Can you work these out from the model? Positions are in its coordinate system, mm. A direction names the side the tool comes from. Coordinates: 2 decimals unless noted, no trailing zeros. Loops run counter-clockwise (first coordinate to the right, second up) from the corner with the lowest first, then second, coordinate; pieces in that order, holes last. Notation, with made-up numbers: (57.25, 1) -> (96.25, 1) arc R20 cw to (96.25, 18) -> close; hole circle Ø5 at (67.5, -1.5). An arc over 180 degrees is marked (long way). Put each result on its own line as item: value. Start each with the question number.
Item 1: We'd pull the mould along Z, two halves only. Please class faces 1 (the flat face through (0, 11, -20.5)), 2 (the cylindrical face through (-41, -73.95, 21.07)), 3 (the cylindrical face through (-41.07, -73.95, -21)): pulls with the +Z half, pulls with the -Z half, needs draft (parallel to the pull), parting line crosses it, or undercut.
Item 2: Will these pins go through, and if not, where does the flat tip stop? P1, Ø0.6, axis at x = 2.5, z = -21, coming from the +Y side; P2, Ø0.6, axis at y = -153.5, z = -21.5, coming from the +X side; P3, Ø22.5, axis at x = 12.5, z = 8, coming from the -Y side.
Item 3: If we section it at B-B on x = -33: Please give me the cut outline in (y, z), plus the area to 3 significant figures.
Item 4: If we section it at D-D on z = -15.5: Please give me the cut outline in (x, y).
Item 5: Please list where these lines run through material, in increasing order: L1, parallel to X at y = -157.5, z = -21.65; L2, parallel to Y at x = 0, z = -21.8; L3, parallel to Y at x = 4, z = 14.5. Write a range as from..to.
Item 6: If we section it at A-A on x = 0: Please give me the cut outline in (y, z), plus the area to 3 significant figures.
Item 7: If we section it at C-C on z = 4: Please give me the cut outline in (x, y).
Item 8: For faces 4 (the cylindrical face through (-5.46, 12.32, 7)), 5 (the flat face through (0, -161, -20.5)), 6 (the flat face through (-1, -76, -22.5)), which set-ups out of +Z, -Z, +X, -X, +Y, -Y let a thin tool reach every point of the face, with its end or its side?
```python
from build123d import *

# Parameters (mm, degrees)
F1_DEPTH = 150
F2_R     = 3
F3_DEPTH = 2
F4_R     = 10
F5_DEPTH = 25


with BuildPart() as f1:
    # F0 (on Front) → F1 (new body)
    with BuildSketch(Plane.XZ):
        with BuildLine():
            ThreePointArc((42.5, 17.5), (41.035534, 21.035534), (37.5, 22.5))
            Line((37.5, 22.5), (-37.5, 22.5))
            ThreePointArc((-37.5, 22.5), (-41.035534, 21.035534), (-42.5, 17.5))
            Line((-42.5, 17.5), (-42.5, -17.5))
            ThreePointArc((-42.5, -17.5), (-41.035534, -21.035534), (-37.5, -22.5))
            Line((-37.5, -22.5), (37.5, -22.5))
            ThreePointArc((37.5, -22.5), (41.035534, -21.035534), (42.5, -17.5))
            Line((42.5, -17.5), (42.5, 17.5))
        make_face()
    extrude(amount=F1_DEPTH)

    # F2 (on face) → F3 (join)
    with BuildSketch(Plane(origin=(0, 0, -22.5), x_dir=(1, 0, 0), z_dir=(0, 0, -1))):
        with BuildLine():
            Line((30, 165), (-30, 165))
            ThreePointArc((-30, 165), (-33.535534, 163.535534), (-35, 160))
            Line((-35, 160), (-35, -10))
            ThreePointArc((-35, -10), (-33.535534, -13.535534), (-30, -15))
            Line((-30, -15), (30, -15))
            ThreePointArc((30, -15), (33.535534, -13.535534), (35, -10))
            Line((35, -10), (35, 160))
            ThreePointArc((35, 160), (33.535534, 163.535534), (30, 165))
        make_face()
        with BuildLine():
            Line((-21, -4.5), (-15, -4.5))
            ThreePointArc((-15, -4.5), (-12.87868, -5.37868), (-12, -7.5))
            ThreePointArc((-12, -7.5), (-12.87868, -9.62132), (-15, -10.5))
            Line((-15, -10.5), (-21, -10.5))
            ThreePointArc((-21, -10.5), (-23.12132, -9.62132), (-24, -7.5))
            ThreePointArc((-24, -7.5), (-23.12132, -5.37868), (-21, -4.5))
        make_face(mode=Mode.SUBTRACT)
        with Locations((0, -7.5)):
            Circle(F2_R, mode=Mode.SUBTRACT)
        with BuildLine():
            ThreePointArc((24, -7.5), (23.12132, -9.62132), (21, -10.5))
            Line((21, -10.5), (15, -10.5))
            ThreePointArc((15, -10.5), (12.87868, -9.62132), (12, -7.5))
            ThreePointArc((12, -7.5), (12.87868, -5.37868), (15, -4.5))
            Line((15, -4.5), (21, -4.5))
            ThreePointArc((21, -4.5), (23.12132, -5.37868), (24, -7.5))
        make_face(mode=Mode.SUBTRACT)
        with BuildLine():
            Line((-21, 160.5), (-15, 160.5))
            ThreePointArc((-15, 160.5), (-12.87868, 159.62132), (-12, 157.5))
            ThreePointArc((-12, 157.5), (-12.87868, 155.37868), (-15, 154.5))
            Line((-15, 154.5), (-21, 154.5))
            ThreePointArc((-21, 154.5), (-23.12132, 155.37868), (-24, 157.5))
            ThreePointArc((-24, 157.5), (-23.12132, 159.62132), (-21, 160.5))
        make_face(mode=Mode.SUBTRACT)
        with Locations((0, 157.5)):
            Circle(F2_R, mode=Mode.SUBTRACT)
        with BuildLine():
            ThreePointArc((12, 157.5), (12.87868, 159.62132), (15, 160.5))
            Line((15, 160.5), (21, 160.5))
            ThreePointArc((21, 160.5), (23.12132, 159.62132), (24, 157.5))
            ThreePointArc((24, 157.5), (23.12132, 155.37868), (21, 154.5))
            Line((21, 154.5), (15, 154.5))
            ThreePointArc((15, 154.5), (12.87868, 155.37868), (12, 157.5))
        make_face(mode=Mode.SUBTRACT)
    extrude(amount=-F3_DEPTH)

    # F4 (on Front) → F5 (join)
    with BuildSketch(Plane.XZ):
        with Locations((15, 4)):
            Circle(F4_R)
        with Locations((-15, 4)):
            Circle(F4_R)
    extrude(amount=-F5_DEPTH)


solid = f1.part
```
Solutions:
1. face 1: undercut
1. face 2: pulls with the +Z half
1. face 3: pulls with the -Z half
2. P1: y = 15
2. P2: x = 35
2. P3: y = -150
3. outline: (-164, -22.5) -> (14, -22.5) -> (14, -20.5) -> (0, -20.5) -> (0, 22.5) -> (-150, 22.5) -> (-150, -20.5) -> (-164, -20.5) -> close
3. area: 6,810 mm^2
4. outline: (-42.5, -150) -> (42.5, -150) -> (42.5, 0) -> (-42.5, 0) -> close
5. L1: -35..-24, -12..-3, 3..12, 24..35
5. L2: -165..-160.5, -154.5..4.5, 10.5..15
5. L3: -150..0
6. outline: (-165, -22.5) -> (-160.5, -22.5) -> (-160.5, -20.5) -> (-165, -20.5) -> close; (-154.5, -22.5) -> (4.5, -22.5) -> (4.5, -20.5) -> (0, -20.5) -> (0, 22.5) -> (-150, 22.5) -> (-150, -20.5) -> (-154.5, -20.5) -> close; (10.5, -22.5) -> (15, -22.5) -> (15, -20.5) -> (10.5, -20.5) -> close
6. area: 6,790 mm^2
7. outline: (-42.5, -150) -> (42.5, -150) -> (42.5, 0) -> (25, 0) -> (25, 25) -> (5, 25) -> (5, 0) -> (-5, 0) -> (-5, 25) -> (-25, 25) -> (-25, 0) -> (-42.5, 0) -> close
8. face 4: +Y
8. face 5: +Z, +X, -X, -Y
8. face 6: -Z, +X, -X, +Y, -Y
